The listing builds one solid part. Answer for the finished solid, in the listing's coordinates (mm). A direction names the side the tool comes from. Round coordinates to 2 decimals unless told otherwise and drop trailing zeros. Write each loop counter-clockwise with the first axis right and the second up, starting at its lowest first coordinate (ties: lowest second). Pieces come first, ordered by that corner, then holes. Notation, with made-up numbers: (68, 16) - (106, 16) arc R20 ccw to (106, 46) - close; hole circle Ø1 at (28.5, 72). An arc over 180 degrees is marked (long way). Return JSON: item names as keys, results as strings. Group by question number.
(1) Find the intervals of material crossed by line 1 along X through (y, z) = (1.8, 76.16); line 2 along X through (y, z) = (2.35, 14); line 3 along Z through (x, y) = (6, 2.1), in increasing order. Write a range as [from, to].
(2) Each of these flat-tipped pins is pushed along its axis until it touches: pin 1 (1.5 mm diameter, centred on x = 11.5, z = 39, fed in from -Y); pin 2 (1.5 mm diameter, centred on y = 1, z = -2.5, fed in from -X). Where does it stop, or does it pass through?
(3) Section A-A, the plane z = 14 is taken. Write down the section's boundary in (x, y).
(4) Determine the mould class of faces 4 (the flat face through (9.554, 1.521, 60.282)), 5 (the cylindrical face through (-18.4, 1.48, 8.14)), 6 (the flat face through (-2, 0, 26)) for opening direction X: +X half, -X half, draft (parallel to the pull), parting line (faces both ways), or undercut.
(5) Section D-D, the plane y = 0.7 is taken. Give the number of separate pieces and of enclosed holes in the cut face, then the cut area to 3 significant figures.
(6) Section B-B, the plane x = -14 is taken. Write down the section's boundary in (y, z).
(7) Section C-C, the plane x = 19.5 is taken. Write down the section's boundary in (y, z), then the cut area to 3 significant figures.
(8) Which of the six approach directions +Z, -Z, +X, -X, +Y, -Y give full straight-line access (tool end or side, diameter ignored) to faces 1 (the flat face through (0, 2, -12)), 2 (the flat face through (0, 2, 26.66)), 3 (the flat face through (-17.5, 2, 0))?
```python
from build123d import *

# Parameters (mm, degrees)
SKETCH_1_W          = 47
SKETCH_1_H          = 40
SKETCH_1_R          = 1.5
SKETCH_1_W_2        = 30
SKETCH_1_H_2        = 12
SKETCH_1_H_3        = 66.16
SKETCH_1_W_3        = 15
EXTRUDE_1_DEPTH     = 3
SKETCH_4_R          = 1.5
SKETCH_4_W          = 47
SKETCH_4_H          = 5
CUT_EXTRUDE_2_DEPTH = 4
SKETCH_7_W          = 30
SKETCH_7_H          = 8
SKETCH_7_W_2        = 6
SKETCH_7_H_2        = 18
CUT_EXTRUDE_3_DEPTH = 10
FILLET_2_R          = 3
FILLET_3_R          = 1
CUT_EXTRUDE_4_DEPTH = 10
FILLET_4_R          = 2
FILLET_5_R          = 5
FILLET_6_R          = 3
FILLET_7_R          = 3


# Some blends are built 0.0001 mm under size
with BuildPart() as part:
    # 草图1 → 凸台-拉伸1 (new body)
    # profile 1 of 3: a face of its own
    with BuildSketch(Plane(origin=(0, 0, 0), x_dir=(1, 0, 0), z_dir=(0, 1, 0))):
        Rectangle(SKETCH_1_W, SKETCH_1_H)
        with Locations(Location((19.5, -14, 0), (0, 0, 270))):
            Circle(SKETCH_1_R, mode=Mode.SUBTRACT)
        with Locations(Location((19.5, 14, 0), (0, 0, 270))):
            Circle(SKETCH_1_R, mode=Mode.SUBTRACT)
        with Locations(Location((-19.5, -14, 0), (0, 0, 270))):
            Circle(SKETCH_1_R, mode=Mode.SUBTRACT)
        with Locations(Location((-19.5, 14, 0), (0, 0, 270))):
            Circle(SKETCH_1_R, mode=Mode.SUBTRACT)
        with Locations((0, -13)):
            Rectangle(SKETCH_1_W_2, SKETCH_1_H_2, mode=Mode.SUBTRACT)
    # profile 2 of 3: a face of its own
    with BuildSketch(Plane(origin=(0, 0, 0), x_dir=(1, 0, 0), z_dir=(0, 1, 0))):
        with Locations((0, -53.08)):
            Rectangle(SKETCH_1_W, SKETCH_1_H_3)
    # profile 3 of 3: a face of its own
    with BuildSketch(Plane(origin=(0, 0, 0), x_dir=(1, 0, 0), z_dir=(0, 1, 0))):
        with Locations((-7.5, -13)):
            Rectangle(SKETCH_1_W_3, SKETCH_1_H_2)
    extrude(amount=EXTRUDE_1_DEPTH)

    # 草图4 → 切除-拉伸2 (cut)
    with BuildSketch(Plane(origin=(0, 3, 0), x_dir=(1, 0, 0), z_dir=(0, 1, 0))):
        with Locations(Location((-14, -76.16, 0), (0, 0, 270))):
            Circle(SKETCH_4_R)
        with Locations(Location((14, -76.16, 0), (0, 0, 270))):
            Circle(SKETCH_4_R)
        with Locations((0, -83.66)):
            Rectangle(SKETCH_4_W, SKETCH_4_H)
    extrude(amount=-CUT_EXTRUDE_2_DEPTH, mode=Mode.SUBTRACT)

    # 草图7 → 切除-拉伸3 (cut)
    with BuildSketch(Plane(origin=(0, 3, 0), x_dir=(1, 0, 0), z_dir=(0, 1, 0))):
        with Locations((0, 16)):
            Rectangle(SKETCH_7_W, SKETCH_7_H)
        with Locations((20.5, 0)):
            Rectangle(SKETCH_7_W_2, SKETCH_7_H_2)
        with Locations((-20.5, 0)):
            Rectangle(SKETCH_7_W_2, SKETCH_7_H_2)
    extrude(amount=-CUT_EXTRUDE_3_DEPTH, mode=Mode.SUBTRACT)

    # 圆角2
    fillet_2_edges = [part.edges().sort_by_distance(p)[0] for p in [
        (-23.5, 1.5, -20),
        (23.5, 1.5, -20),
    ]]
    fillet(fillet_2_edges, radius=FILLET_2_R)

    # 圆角3
    fillet_3_edges = [part.edges().sort_by_distance(p)[0] for p in [
        (0, 1.5, 19),
        (15, 1.5, 19),
        (15, 1.5, 7),
        (0, 1.5, 7),
    ]]
    fillet(fillet_3_edges, radius=FILLET_3_R)

    # 草图9 → 切除-拉伸4 (cut)
    with BuildSketch(Plane(origin=(0, 3, 0), x_dir=(1, 0, 0), z_dir=(0, 1, 0))):
        Polygon((-3, -49.16), (-16.258928571, -26.66), (-18.5, -26.66), (-18.5, -71.66), (-16.258928571, -71.66), align=None)
        Polygon((0, -47.16), (12.080357143, -26.66), (-12.080357143, -26.66), align=None)
        Polygon((18.5, -26.66), (16.258928571, -26.66), (3, -49.16), (16.258928571, -71.66), (18.5, -71.66), align=None)
        Polygon((-12.080357143, -71.66), (12.080357143, -71.66), (0, -51.16), align=None)
    extrude(amount=-CUT_EXTRUDE_4_DEPTH, mode=Mode.SUBTRACT)

    # 圆角4
    # the kernel refuses this fillet: 2 mm, written as the material it adds along each edge
    with BuildSketch(Plane(origin=(16.258928571, 3, 71.66), x_dir=(-0.5076923076923154, 0, -0.8615384615384569), z_dir=(0, -1, 0)), Plane(origin=(16.258928571, 3, 26.66), x_dir=(1, 0, 0), z_dir=(0, -1, 0)), Plane(origin=(-16.258928571, 3, 71.66), x_dir=(-1, 0, 0), z_dir=(0, -1, 0)), Plane(origin=(-16.258928571, 3, 26.66), x_dir=(0.5076923076923154, 0, 0.8615384615384569), z_dir=(0, -1, 0))) as fillet_4_piece_1:
        with BuildLine():
            CenterArc((FILLET_4_R * 0.571428571429, FILLET_4_R), FILLET_4_R, 210.510237406, 59.489762594)
            Line((-FILLET_4_R * 0.29010989011, FILLET_4_R * 0.492307692308), (0, 0))
            Line((0, 0), (FILLET_4_R * 0.571428571429, 0))
        make_face()
    extrude(amount=3)
    with BuildSketch(Plane(origin=(3, 3, 49.16), x_dir=(0.5076923076923108, 0, -0.8615384615384596), z_dir=(0, -1, 0))) as fillet_4_piece_2:
        with BuildLine():
            CenterArc((FILLET_4_R * 0.589285714286, FILLET_4_R), FILLET_4_R, 208.979525188, 61.020474812)
            Line((-FILLET_4_R * 0.285507185123, FILLET_4_R * 0.51550295858), (0, 0))
            Line((0, 0), (FILLET_4_R * 0.589285714286, 0))
        make_face()
    extrude(amount=3)
    with BuildSketch(Plane(origin=(18.5, 3, 26.66), x_dir=(-1, 0, 0), z_dir=(0, -1, 0))) as fillet_4_piece_3:
        with BuildLine():
            CenterArc((FILLET_4_R, -FILLET_4_R), FILLET_4_R, 90, 90)
            Line((0, -FILLET_4_R), (0, 0))
            Line((0, 0), (FILLET_4_R, 0))
        make_face()
    extrude(amount=3)
    with BuildSketch(Plane(origin=(18.5, 3, 71.66), x_dir=(-1, 0, 0), z_dir=(0, -1, 0)), Plane(origin=(-18.5, 3, 71.66), x_dir=(0, 0, -1), z_dir=(0, -1, 0)), Plane(origin=(-18.5, 3, 26.66), x_dir=(1, 0, 0), z_dir=(0, -1, 0))) as fillet_4_piece_4:
        with BuildLine():
            CenterArc((FILLET_4_R, FILLET_4_R), FILLET_4_R, 180, 90)
            Line((0, FILLET_4_R), (0, 0))
            Line((0, 0), (FILLET_4_R, 0))
        make_face()
    extrude(amount=3)
    with BuildSketch(Plane(origin=(-12.080357143, 3, 26.66), x_dir=(0.5076923076923134, 0, 0.8615384615384581), z_dir=(0, -1, 0)), Plane(origin=(-12.080357143, 3, 71.66), x_dir=(1, 0, 0), z_dir=(0, -1, 0))) as fillet_4_piece_5:
        with BuildLine():
            CenterArc((FILLET_4_R * 1.75, -FILLET_4_R), FILLET_4_R, 90, 120.510237406)
            Line((FILLET_4_R * 0.888461538462, -FILLET_4_R * 1.50769230769), (0, 0))
            Line((0, 0), (FILLET_4_R * 1.75, 0))
        make_face()
    extrude(amount=3)
    with BuildSketch(Plane(origin=(12.080357143, 3, 26.66), x_dir=(-0.5076923076923134, 0, 0.8615384615384581), z_dir=(0, -1, 0)), Plane(origin=(12.080357143, 3, 71.66), x_dir=(-1, 0, 0), z_dir=(0, -1, 0))) as fillet_4_piece_6:
        with BuildLine():
            CenterArc((FILLET_4_R * 1.75, FILLET_4_R), FILLET_4_R, 149.489762594, 120.510237406)
            Line((FILLET_4_R * 0.888461538462, FILLET_4_R * 1.50769230769), (0, 0))
            Line((0, 0), (FILLET_4_R * 1.75, 0))
        make_face()
    extrude(amount=3)
    with BuildSketch(Plane(origin=(0, 3, 47.16), x_dir=(-0.5076923076923119, 0, -0.8615384615384591), z_dir=(0, -1, 0)), Plane(origin=(0, 3, 51.16), x_dir=(0.5076923076923116, 0, 0.8615384615384594), z_dir=(0, -1, 0))) as fillet_4_piece_7:
        with BuildLine():
            CenterArc((FILLET_4_R * 1.69696969697, FILLET_4_R), FILLET_4_R, 151.020474812, 118.979525188)
            Line((FILLET_4_R * 0.822176797561, FILLET_4_R * 1.48449704142), (0, 0))
            Line((0, 0), (FILLET_4_R * 1.69696969697, 0))
        make_face()
    extrude(amount=3)
    with BuildSketch(Plane(origin=(-3, 3, 49.16), x_dir=(-0.507692307692313, 0, -0.8615384615384584), z_dir=(0, -1, 0))) as fillet_4_piece_8:
        with BuildLine():
            CenterArc((FILLET_4_R * 0.589285714286, -FILLET_4_R), FILLET_4_R, 90, 61.020474812)
            Line((-FILLET_4_R * 0.285507185123, -FILLET_4_R * 0.51550295858), (0, 0))
            Line((0, 0), (FILLET_4_R * 0.589285714286, 0))
        make_face()
    extrude(amount=3)

    # 圆角5
    fillet_5_edges = [part.edges().sort_by_distance(p)[0] for p in [
        (-23.5, 1.5, 81.16),
        (23.5, 1.5, 81.16),
    ]]
    fillet(fillet_5_edges, radius=FILLET_5_R)

    # 圆角6
    fillet_6_edges = [part.edges().sort_by_distance(p)[0] for p in [
        (15, 1.5, -20),
        (15, 1.5, -12),
        (-15, 1.5, -12),
        (-15, 1.5, -20),
        (17.5, 1.5, -9),
        (17.5, 1.5, 9),
        (-17.5, 1.5, 9),
        (-17.5, 1.5, -9),
    ]]
    fillet(fillet_6_edges, radius=FILLET_6_R)

    # 圆角7
    fillet_7_edges = [part.edges().sort_by_distance(p)[0] for p in [
        (23.5, 1.5, -9),
        (23.5, 1.5, 9),
        (-23.5, 1.5, 9),
        (-23.5, 1.5, -9),
    ]]
    fillet(fillet_7_edges, radius=FILLET_7_R - 0.0001)  # a hair under: the kernel refuses the full size


solid = part.part
```
Working result:
{
 "1": {"line 1": "x = [-23.5, -15.5], [-12.5, 12.5], [15.5, 23.5]", "line 2": "x = [-23.5, -21], [-18, 0], [15, 18], [21, 23.5]", "line 3": "z = [-12, 7], [19, 26.66], [36.98, 44.07], [54.25, 61.34], [71.66, 81.16]"},
 "2": {"pin 1": "passes through", "pin 2": "stops at x = -17.5"},
 "3": {"outline": "(-23.5, 0) - (-21, 0) - (-21, 3) - (-23.5, 3) - close; (-18, 0) - (0, 0) - (0, 3) - (-18, 3) - close; (15, 0) - (18, 0) - (18, 3) - (15, 3) - close; (21, 0) - (23.5, 0) - (23.5, 3) - (21, 3) - close"},
 "4": {"face 4": "undercut", "face 5": "-X half", "face 6": "draft"},
 "5": {"separate pieces": "1", "enclosed holes": "11", "area": "2,790 mm^2"},
 "6": {"outline": "(0, -12.76) - (3, -12.76) - (3, 30.49) - (0, 30.49) - close; (0, 67.83) - (3, 67.83) - (3, 74.66) - (0, 74.66) - close; (0, 77.66) - (3, 77.66) - (3, 81.16) - (0, 81.16) - close"},
 "7": {"outline": "(0, -20) - (3, -20) - (3, -15.5) - (0, -15.5) - close; (0, -12.5) - (3, -12.5) - (3, -8.83) - (0, -8.83) - close; (0, 8.83) - (3, 8.83) - (3, 12.5) - (0, 12.5) - close; (0, 15.5) - (3, 15.5) - (3, 81.06) - (0, 81.06) - close", "area": "232 mm^2"},
 "8": {"face 1": "-Z, +Y, -Y", "face 2": "+Y, -Y", "face 3": "-X, +Y, -Y"}
}
